```python
from build123d import *

# Parameters (mm, degrees)
SKETCH3_W          = 4.037166667
SKETCH3_H          = 4.037166667
CUT_EXTRUDE1_DEPTH = 38.455371645


with BuildPart() as part:
    # Sweep1: sweep along a path in Sketch2
    with BuildLine(Plane(origin=(0, 0, 0), x_dir=(1, 0, 0), z_dir=(0, 1, 0))) as sweep1_path:
        Line((0, 0), (0, -19.05))
        Line((0, -19.05), (-19.05, -19.05))
    # Sketch1 → Sweep1 (sweep)
    with BuildSketch(Plane.XY):
        Polygon((2.31775, -19.05), (4.31775, -19.05), (4.31775, 2), (-4.31775, 2), (-3.18725, -22.225), (-1.280583333, -22.225), (-2.31775, 0), (2.31775, 0), align=None)
    sweep(path=sweep1_path.line, transition=Transition.RIGHT)

    # Sketch3 → Cut-Extrude1 (cut, through all)
    with BuildSketch(Plane.XZ):
        with Locations((-3.299166667, 15.750833334)):
            Rectangle(SKETCH3_W, SKETCH3_H)
    extrude(amount=CUT_EXTRUDE1_DEPTH, mode=Mode.SUBTRACT)


solid = part.part
```
Source: CAD feature listing. Evaluate the final solid. Frame: model axes, mm. A direction names the side the tool comes from. Round coordinates to 2 decimals unless told otherwise and drop trailing zeros. Loops run counter-clockwise (first coordinate to the right, second up) from the corner with the lowest first, then second, coordinate; pieces in that order, holes last. Notation, with made-up numbers: M -10,63.25 L 29,63.25 A31 cw 29,88.25 Z; hole C 3,38 d6. An arc over 180 degrees is marked long. Use a Markdown table: item, result. Add a question column.
1. Cut plane D-D, the plane x = -12.75. Output: boundary loops of the cut face in (y, z) (3 decimals).
2. Contact query for flat-ended pins moving along their axis: pin 1 (10 mm diameter, centred on x = -6.5, z = 7, fed in from +Y); pin 2 (6 mm diameter, centred on x = -11.5, z = 9.5, fed in from -Y); pin 3 (10 mm diameter, centred on y = -13, z = 5.5, fed in from -X). Output: stop coordinate, or through.
3. Ray query, line 1 along X through (y, z) = (-6, 15.25); line 2 along Z through (x, y) = (-11.75, -8.75); line 3 along Y through (x, z) = (0.25, 20.5). Return the intervals inside material, ascending. Write a range as [from, to].
4. Set-up query: faces 5 (the flat face through (-5.318, -11, 16)), 6 (the flat face through (-3, -11, 13.732)), 7 (the flat face through (-2, -19.05, 22)). Return all of +Z, -Z, +X, -X, +Y, -Y with unobstructed straight access to the full face (end or side cutting, diameter ignored); none if empty.
5. Cut plane B-B, the plane x = -2.75. Output: boundary loops of the cut face in (y, z) (3 decimals), and give its area (3 significant figures).
6. Pull-direction query (Z, two-part tool) for faces 1 (the flat face through (-12, -22.225, 17)), 2 (the flat face through (-4, 0, 16)), 3 (the flat face through (-11.74, -9.94, 15.29)), 4 (the flat face through (-8, -9, 23.368)); classes: +Z half, -Z half, draft (parallel to the pull), parting line (faces both ways), or undercut.
7. Cut plane C-C, the plane z = 19.75. Output: boundary loops of the cut face in (x, y), and give its area (3 significant figures).
8. Cut plane A-A, the plane y = -17.25. Output: boundary loops of the cut face in (x, z).
Solution:
| question | item | result |
|---|---|---|
| 1 | outline | M -22.225,15.863 L 2,14.732 L 2,23.368 L -19.05,23.368 L -19.05,21.368 L 0,21.368 L 0,16.732 L -22.225,17.769 Z |
| 2 | pin 1 | stops at y = 2 |
| 2 | pin 2 | passes through |
| 2 | pin 3 | stops at x = -3.85 |
| 3 | line 1 | x = [-19.05, -5.32], [2.32, 4.32] |
| 3 | line 2 | z = [15.23, 17.14], [21.37, 23.37] |
| 3 | line 3 | y = [0, 2] |
| 4 | face 5 | -Z, -Y |
| 4 | face 6 | -X, -Y |
| 4 | face 7 | +Z, +X, -Y |
| 5 | outline | M -22.225,0 L 2,0 L 2,23.368 L -19.05,23.368 L -19.05,21.368 L 0,21.368 L 0,13.732 L -22.225,13.732 Z |
| 5 | area | 390 mm2 |
| 6 | face 1 | draft |
| 6 | face 2 | undercut |
| 6 | face 3 | -Z half |
| 6 | face 4 | +Z half |
| 7 | outline | M -19.05,0 L 2.32,0 L 2.32,-19.05 L 4.32,-19.05 L 4.32,2 L -19.05,2 Z |
| 7 | area | 84.8 mm2 |
| 8 | outline | M -19.05,15.63 L -5.32,15.63 L -5.32,17.54 L -19.05,17.54 Z; M -19.05,21.37 L 2.32,21.37 L 2.32,0 L 4.32,0 L 4.32,23.37 L -19.05,23.37 Z; M -3.42,0 L -1.51,0 L -1.51,13.73 L -3.42,13.73 Z |
